```python
from build123d import *

# Parameters (mm, degrees)
F0_W     = 335
F0_H     = 734
F1_DEPTH = 408
F2_W     = 198
F2_H     = 198
F3_DEPTH = 300


with BuildPart() as f1:
    # F0 (on Right) → F1 (new body)
    with BuildSketch(Plane.YZ):
        with Locations((-3.853569, 367)):
            Rectangle(F0_W, F0_H)
    extrude(amount=-F1_DEPTH)

    # F2 (on face) → F3 (join)
    with BuildSketch(Plane.YZ):
        with Locations((-3.853569, 288)):
            Rectangle(F2_W, F2_H)
    extrude(amount=F3_DEPTH)


solid = f1.part
```
CAD build for the part. Positions are in the model's coordinates, mm. A direction names the side the tool comes from. Coordinates: 2 decimals unless noted, no trailing zeros. Write each loop counter-clockwise with the first axis right and the second up, starting at its lowest first coordinate (ties: lowest second). Pieces come first, ordered by that corner, then holes.
(1) Drill centre lines: probe 1 along X at (y, z) = (126, 165.5); probe 2 along Z at (x, y) = (263, -33.5); probe 3 along Y at (x, z) = (262, 301.5). Where is each one in solid material? Low to high.
(2) Flat gauge pins, fed straight in: pin 1 (8 mm diameter, centred on x = 23, z = 243.5, fed in from +Y); pin 2 (12 mm diameter, centred on y = 12.5, z = 399, fed in from +X). Where does each tip first touch, or does it go through?
(3) Cut at B-B, the plane y = -66.5. List the corners of the cut face in (x, z), and give its area (3 significant figures).
(4) 3-axis set-ups, long thin cutter, end or side, ignore diameter. For faces 1 (the face through (148, -5, 387)), 2 (the face through (148, -5, 189)), 3 (the face through (148, 95.146, 287)): which of +Z, -Z, +X, -X, +Y, -Y reach the whole face in a straight line?
(5) Cut at C-C, the plane x = 105. List the corners of the cut face in (y, z).
(6) Cut at A-A, the plane z = 356. List the corners of the cut face in (x, y), and give its area (3 significant figures).
(7) Cut at D-D, the plane z = 438. List the corners of the cut face in (x, y).
Geometry says:
1. probe 1: x = -408 to 0
1. probe 2: z = 189 to 387
1. probe 3: y = -102.85 to 95.15
2. pin 1: stops at y = 95.15
2. pin 2: stops at x = 0
3. outline: (-408, 0) - (0, 0) - (0, 189) - (300, 189) - (300, 387) - (0, 387) - (0, 734) - (-408, 734) - close
3. area: 359,000 mm2
4. face 1: +Z, +X, +Y, -Y
4. face 2: -Z, +X, +Y, -Y
4. face 3: +Z, -Z, +X, +Y
5. outline: (-102.85, 189) - (95.15, 189) - (95.15, 387) - (-102.85, 387) - close
6. outline: (-408, -171.35) - (0, -171.35) - (0, -102.85) - (300, -102.85) - (300, 95.15) - (0, 95.15) - (0, 163.65) - (-408, 163.65) - close
6. area: 196,000 mm2
7. outline: (-408, -171.35) - (0, -171.35) - (0, 163.65) - (-408, 163.65) - close
